The figure shows three views and two pictorial views of one solid part (mm, origin at its lowest corner). Answer the questions. A direction names the side the tool comes from. Coordinates: 2 decimals unless noted, no trailing zeros. Loops run counter-clockwise (first coordinate to the right, second up) from the corner with the lowest first, then second, coordinate; pieces in that order, holes last. Notation, with made-up numbers: M 34,-19.75 L 71,-19.75 A30 cw 71,2.25 Z; hole C 74,-2 d9. An arc over 180 degrees is marked long. Return JSON: item names as keys, results as strings. Group by question number.
1. Section A-A (x = 5) is taken. Write down the section's boundary in (y, z), then the cut area to 3 significant figures.
2. Which of the six approach directions +Z, -Z, +X, -X, +Y, -Y give full straight-line access (tool end or side, diameter ignored) to the marked faces 5, 6 and 7?
3. The mould has two halves that part along Y. Classify the marked faces 1, 2, 3 and 4: pulls with the +Y half, pulls with the -Y half, needs draft (parallel to the pull), parting line crosses it, or undercut.
4. Given P1, Ø2, axis at x = 5.5, y = 16, coming from the +Z side; P2, Ø2, axis at x = 6.5, y = 7, coming from the +Z side; P3, Ø1.6, axis at x = 2.5, y = 20, coming from the +Z side, each flat-ended and moving along its own axis, determine where each tip first touches the part or whether it passes through.
5. Section B-B (z = 3) is taken. Write down the section's boundary in (x, y).
6. Straight lines are drawn through the part: L1, parallel to Y at x = 3.5, z = 6.5; L2, parallel to X at y = 1.4, z = 8.4; L3, parallel to Z at x = 8, y = 7.25. For each, find the intervals that lie inside material, in ascending order. Write a range as from..to.
7. Section C-C (z = 8.4) is taken. Write down the section's boundary in (x, y), then the cut area to 3 significant figures.
8. Section D-D (x = 2.5) is taken. Write down the section's boundary in (y, z).
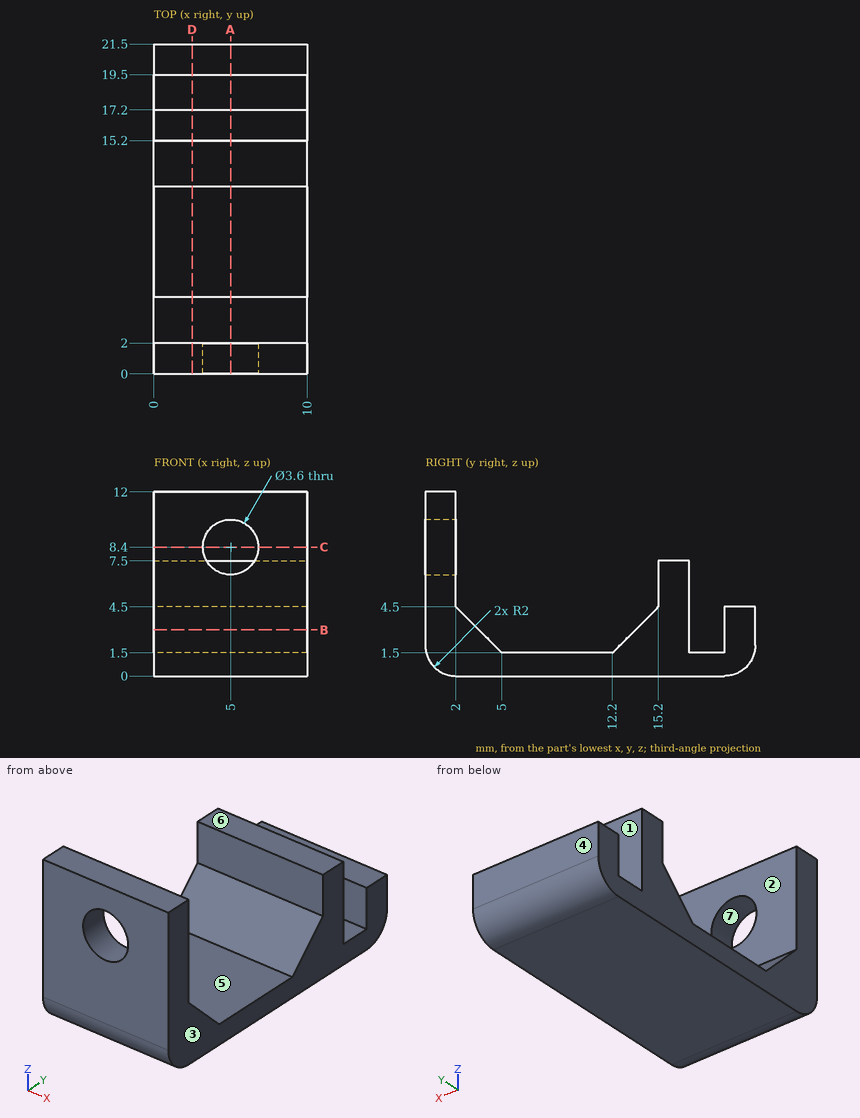
Worked out:
{
 "1": {"outline": "M 0,2 A2 ccw 2,0 L 19.5,0 A2 ccw 21.5,2 L 21.5,4.5 L 19.5,4.5 L 19.5,1.5 L 17.2,1.5 L 17.2,7.5 L 15.2,7.5 L 15.2,4.5 L 12.2,1.5 L 5,1.5 L 2,4.5 L 2,6.6 L 0,6.6 Z; M 0,10.2 L 2,10.2 L 2,12 L 0,12 Z", "area": "71.3 mm^2"},
 "2": {"face 5": "+Z, +X, -X", "face 6": "+Z, +X, -X, +Y", "face 7": "-Y"},
 "3": {"face 1": "undercut", "face 2": "undercut", "face 3": "needs draft", "face 4": "pulls with the +Y half"},
 "4": {"P1": "z = 7.5", "P2": "z = 1.5", "P3": "z = 4.5"},
 "5": {"outline": "M 0,0 L 10,0 L 10,3.5 L 0,3.5 Z; M 0,13.7 L 10,13.7 L 10,17.2 L 0,17.2 Z; M 0,19.5 L 10,19.5 L 10,21.5 L 0,21.5 Z"},
 "6": {"L1": "0..2, 15.2..17.2", "L2": "0..3.2, 6.8..10", "L3": "0..1.5"},
 "7": {"outline": "M 0,0 L 3.2,0 L 3.2,2 L 0,2 Z; M 6.8,0 L 10,0 L 10,2 L 6.8,2 Z", "area": "12.8 mm^2"},
 "8": {"outline": "M 0,2 A2 ccw 2,0 L 19.5,0 A2 ccw 21.5,2 L 21.5,4.5 L 19.5,4.5 L 19.5,1.5 L 17.2,1.5 L 17.2,7.5 L 15.2,7.5 L 15.2,4.5 L 12.2,1.5 L 5,1.5 L 2,4.5 L 2,12 L 0,12 Z"}
}
